Design review of the part built by this model. Coordinates are the model's own, in mm. Coordinates: 2 decimals unless noted, no trailing zeros. Order: outer loops, then holes, each group sorted by start corner. A loop starts at its lowest first (then second) coordinate and runs counter-clockwise, first axis right, second up.
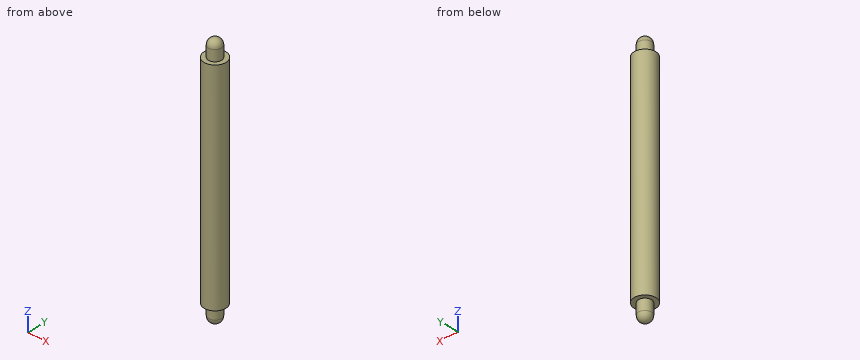
from build123d import *

# Parameters (mm, degrees)
SKETCH1_R           = 5
BOSS_EXTRUDE1_DEPTH = 100
SKETCH2_R           = 3
BOSS_EXTRUDE2_DEPTH = 8
SKETCH4_R           = 3
BOSS_EXTRUDE3_DEPTH = 8
FILLET1_R           = 3


with BuildPart() as part:
    # Sketch1 → Boss-Extrude1 (new body)
    with BuildSketch(Plane.XY):
        with Locations((-48.10405297, 10.230555556)):
            Circle(SKETCH1_R)
    extrude(amount=BOSS_EXTRUDE1_DEPTH)

    # Sketch2 → Boss-Extrude2 (add)
    with BuildSketch(Plane.XY.offset(100)):
        with Locations((-48.10405297, 10.230555556)):
            Circle(SKETCH2_R)
    extrude(amount=BOSS_EXTRUDE2_DEPTH)

    # Sketch4 → Boss-Extrude3 (add)
    with BuildSketch(Plane(origin=(0, 0, 0), x_dir=(-1, 0, 0), z_dir=(0, 0, -1))):
        with Locations((48.10405297, 10.230555556)):
            Circle(SKETCH4_R)
    extrude(amount=BOSS_EXTRUDE3_DEPTH)

    # Fillet1
    fillet1_edges = [part.edges().sort_by_distance(p)[0] for p in [
        (-45.10405297, 10.230555556, -8),
        (-51.10405297, 10.230555556, 108),
    ]]
    fillet(fillet1_edges, radius=FILLET1_R)


solid = part.part
1. Add section C-C (z = 34). Give the boundary of the cut face in (x, y).
2. Insertion check: pin 1 (2 mm diameter, centred on y = 7.5, z = 86.5, fed in from -X) (3 decimals); pin 2 (3 mm diameter, centred on y = 6.5, z = 64.5, fed in from -X); pin 3 (5 mm diameter, centred on x = -44.5, z = 26.5, fed in from +Y). Each pin has a flat end and moves straight along its axis. Give the tip position at first contact, or say it passes through.
3. To check wall thickness, follow line 1 (X direction, y = 10, z = 29); line 2 (Z direction, x = -44.25, y = 11); line 3 (Y direction, x = -45, z = 49.5). State the ranges of each line that lie inside material, in increasing order.
4. Add section B-B (x = -46.25). Give the boundary of the cut face in (y, z), and give its area (3 significant figures).
5. Add section A-A (y = 8.75). Give the boundary of the cut face in (x, z).
Solution:
1. outline: circle Ø10 at (-48.1, 10.23)
2. pin 1: stops at x = -52.795
2. pin 2: stops at x = -52.58
2. pin 3: stops at y = 15.11
3. line 1: x = -53.1 to -43.11
3. line 2: z = 0 to 100
3. line 3: y = 6.31 to 14.15
4. outline: (5.59, 0) - (7.87, 0) - (7.87, -5) arc R2.36 ccw to (12.59, -5) - (12.59, 0) - (14.87, 0) - (14.87, 100) - (12.59, 100) - (12.59, 105) arc R2.36 ccw to (7.87, 105) - (7.87, 100) - (5.59, 100) - close
4. area: 993 mm2
5. outline: (-52.88, 0) - (-50.71, 0) - (-50.71, -5) arc R2.61 ccw to (-45.49, -5) - (-45.49, 0) - (-43.33, 0) - (-43.33, 100) - (-45.49, 100) - (-45.49, 105) arc R2.61 ccw to (-50.71, 105) - (-50.71, 100) - (-52.88, 100) - close
